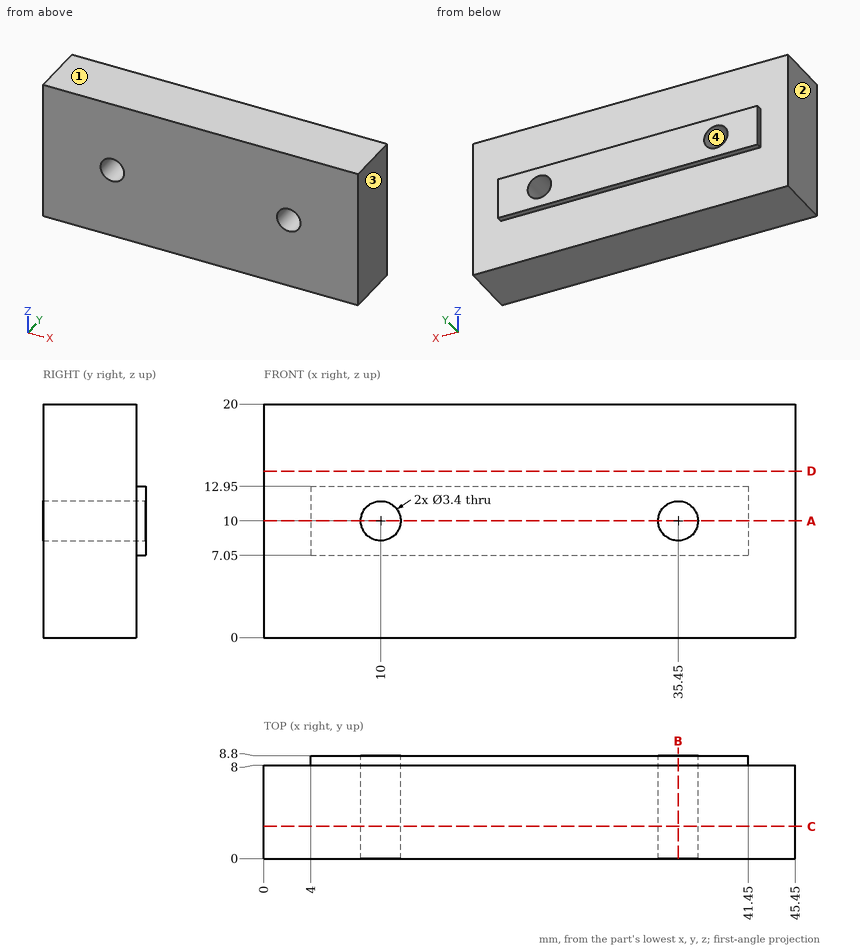
Job drawing, mm, ordinate dimensions from the low corner. One solid piece. Give positions to 0.01 mm unless a question says otherwise; leave off trailing zeros. Loops run counter-clockwise (first coordinate to the right, second up) from the corner with the lowest first, then second, coordinate; pieces in that order, holes last. Notation, with made-up numbers: (-1, 13.25) -> (15, 13.25) arc R12 ccw to (15, 31.25) -> close; hole circle Ø3 at (-23.5, 80). An arc over 180 degrees is marked (long way). Use a Markdown table: item, result. Add a question column.
(1) Slice it at B-B on x = 35.45. List the corners of the cut face in (y, z), and give its area (3 significant figures).
(2) Slice it at A-A on z = 10. List the corners of the cut face in (x, y), and give its area (3 significant figures).
(3) Drop a flat-ended pin along its axis: pin 1 Ø0.9 at (y, z) = (8.5, 10.5) entering from -X. Give the stop position or say it passes through.
(4) Slice it at C-C on y = 2.75. List the corners of the cut face in (x, z).
(5) Mould opens along X. For the marked faces 1, 2, 3 and 4 say: +X half, -X half, draft (parallel to the pull), parting line (faces both ways), or undercut.
(6) Wall check: line 1 along X through (y, z) = (4.75, 10); line 2 along X through (y, z) = (7.5, 11.25); line 3 along Y through (x, z) = (10, 16.5). Give the ranges that are in metal, low to high.
(7) Slice it at D-D on z = 14.25. List the corners of the cut face in (x, y).
Filled sheet:
| question | item | result |
|---|---|---|
| 1 | outline | (0, 0) -> (8, 0) -> (8, 7.05) -> (8.8, 7.05) -> (8.8, 8.3) -> (0, 8.3) -> close; (0, 11.7) -> (8.8, 11.7) -> (8.8, 12.95) -> (8, 12.95) -> (8, 20) -> (0, 20) -> close |
| 1 | area | 135 mm2 |
| 2 | outline | (0, 0) -> (8.3, 0) -> (8.3, 8.8) -> (4, 8.8) -> (4, 8) -> (0, 8) -> close; (11.7, 0) -> (33.75, 0) -> (33.75, 8.8) -> (11.7, 8.8) -> close; (37.15, 0) -> (45.45, 0) -> (45.45, 8) -> (41.45, 8) -> (41.45, 8.8) -> (37.15, 8.8) -> close |
| 2 | area | 334 mm2 |
| 3 | pin 1 | x = 4 |
| 4 | outline | (0, 0) -> (45.45, 0) -> (45.45, 20) -> (0, 20) -> close; hole circle Ø3.4 at (10, 10); hole circle Ø3.4 at (35.45, 10) |
| 5 | face 1 | draft |
| 5 | face 2 | -X half |
| 5 | face 3 | +X half |
| 5 | face 4 | undercut |
| 6 | line 1 | 0 to 8.3, 11.7 to 33.75, 37.15 to 45.45 |
| 6 | line 2 | 0 to 8.85, 11.15 to 34.3, 36.6 to 45.45 |
| 6 | line 3 | 0 to 8 |
| 7 | outline | (0, 0) -> (45.45, 0) -> (45.45, 8) -> (0, 8) -> close |
